```python
from build123d import *

# Parameters (mm, degrees)
SKETCH1_R               = 11
BOSS_EXTRUDE1_DEPTH     = 216.66667
BOSS_EXTRUDE2_START     = 216.66667
SKETCH2_R               = 6.8
BOSS_EXTRUDE2_DEPTH     = 19.8
CUT_EXTRUDE2_START      = -1.4
SKETCH4_R               = 0.5
CUT_EXTRUDE2_DEPTH      = 9
SKETCH6_R               = 7
CUT_EXTRUDE3_DEPTH      = 20
CUT_EXTRUDE4_DEPTH      = 237.977817671
CUT_EXTRUDE4_DEPTH_BACK = 237.977817671
SKETCH7_R               = 0.5
CUT_EXTRUDE5_DEPTH      = 237.97781768
CUT_EXTRUDE5_DEPTH_BACK = 237.97781768
SKETCH10_R              = 0.5
CUT_EXTRUDE6_DEPTH      = 237.97781768
CUT_EXTRUDE6_DEPTH_BACK = 237.97781768
SKETCH11_W              = 2
SKETCH11_H              = 46.680194511
BOSS_EXTRUDE3_START     = 2.5
SKETCH14_R              = 10
BOSS_EXTRUDE3_DEPTH     = 28.5


with BuildPart() as part:
    # Sketch1 → Boss-Extrude1 (new body)
    with BuildSketch(Plane(origin=(0, 0, 0), x_dir=(1, 0, 0), z_dir=(0, 1, 0))):
        with Locations(Location((0, 0, 0), (0, 0, 270))):
            Circle(SKETCH1_R)
    extrude(amount=BOSS_EXTRUDE1_DEPTH)

    # Sketch2 → Boss-Extrude2 (add)
    with BuildSketch(Plane(origin=(0, 0, 0), x_dir=(1, 0, 0), z_dir=(0, 1, 0)).offset(BOSS_EXTRUDE2_START)):
        with Locations(Location((0, 0, 0), (0, 0, 90))):
            Circle(SKETCH2_R)
    extrude(amount=BOSS_EXTRUDE2_DEPTH)

    # Sketch4 → Cut-Extrude2 (cut)
    with BuildSketch(Plane(origin=(0, 0, 0), x_dir=(0, 0, -1), z_dir=(1, 0, 0)).offset(CUT_EXTRUDE2_START)):
        with Locations((0, 226.66667)):
            Circle(SKETCH4_R)
    cut_extrude2 = extrude(amount=-CUT_EXTRUDE2_DEPTH, mode=Mode.SUBTRACT)

    # Mirror2: Cut-Extrude2 across plane
    add(cut_extrude2.mirror(Plane(origin=(0, 0, 0), x_dir=(0, 0, 1), z_dir=(1, 0, 0))), mode=Mode.SUBTRACT)

    # Sketch6 → Cut-Extrude3 (cut)
    with BuildSketch(Plane(origin=(0, 0, 0), x_dir=(1, 0, 0), z_dir=(0, 1, 0))):
        with Locations(Location((0, 0, 0), (0, 0, 270))):
            Circle(SKETCH6_R)
    extrude(amount=CUT_EXTRUDE3_DEPTH, mode=Mode.SUBTRACT)

    # Sketch7 → Cut-Extrude4 (cut, two sides: drawn at the far end of the back side and taken through both)
    with BuildSketch(Plane(origin=(0, 0, 0), x_dir=(0, 0, -1), z_dir=(1, 0, 0)).offset(-CUT_EXTRUDE4_DEPTH_BACK)):
        with Locations((0, 10)):
            Circle(SKETCH7_R)
    extrude(amount=CUT_EXTRUDE4_DEPTH + CUT_EXTRUDE4_DEPTH_BACK, mode=Mode.SUBTRACT)

    # Sketch10 → Cut-Extrude5 (cut, two sides: drawn at the far end of the back side and taken through both)
    with BuildSketch(Plane.XY.offset(-CUT_EXTRUDE5_DEPTH_BACK)):
        with Locations((0, 5)):
            Circle(SKETCH10_R)
    extrude(amount=CUT_EXTRUDE5_DEPTH + CUT_EXTRUDE5_DEPTH_BACK, mode=Mode.SUBTRACT)

    # Sketch11 → Cut-Extrude6 (cut, two sides: drawn at the far end of the back side and taken through both)
    with BuildSketch(Plane.XY.offset(-CUT_EXTRUDE6_DEPTH_BACK)):
        with Locations((0, 213.126572745)):
            Rectangle(SKETCH11_W, SKETCH11_H)
    extrude(amount=CUT_EXTRUDE6_DEPTH + CUT_EXTRUDE6_DEPTH_BACK, mode=Mode.SUBTRACT)

    # Sketch14 → Boss-Extrude3 (add)
    with BuildSketch(Plane(origin=(0, 0, 0), x_dir=(0, 0, -1), z_dir=(1, 0, 0)).offset(BOSS_EXTRUDE3_START)):
        with Locations(Location((0, 160, 0), (0, 0, 180))):
            Circle(SKETCH14_R)
    boss_extrude3 = extrude(amount=BOSS_EXTRUDE3_DEPTH)

    # Mirror3: Boss-Extrude3 across plane
    add(boss_extrude3.mirror(Plane(origin=(0, 0, 0), x_dir=(0, 0, 1), z_dir=(1, 0, 0))))


solid = part.part
```
Input: part model. Units: mm. Frame: model coordinates. A direction names the side the tool comes from. Give positions to 0.01 mm unless a question says otherwise; leave off trailing zeros. Order: outer loops, then holes, each group sorted by start corner. A loop starts at its lowest first (then second) coordinate and runs counter-clockwise, first axis right, second up. Notation, with made-up numbers: M 80,5.25 L 124,5.25 A14 cw 124,26.25 Z; hole C 89.5,60 d7. An arc over 180 degrees is marked long. Return JSON: item names as keys, results as strings.
1) Section query D-D on y = 84. Output: boundary loops of the cut face in (x, z).
Taken from the geometry:
{"outline": "C 0,0 d22"}
2) Section query B-B on y = 213.5. Output: boundary loops of the cut face in (x, z).
Taken from the geometry:
{"outline": "M -1,-10.95 L -1,10.95 A11 ccw Z; M 1,-10.95 A11 ccw 1,10.95 Z"}
3) Line query: L1, parallel to Z at x = 0, y = 11.75; L2, parallel to Y at x = -8, z = 0; L3, parallel to Y at x = -5.2, z = 0. Output: solid intervals per line, ascending. Write a range as [from, to].
Taken from the geometry:
{"L1": "z = [-11, -7], [7, 11]", "L2": "y = [0, 9.5], [10.5, 216.67]", "L3": "y = [20, 226.17], [227.17, 236.47]"}
4) Mould query, pull axis X, two halves, no side actions, for faces 4 (the face through (-4.213, 106.817, 10.161)), 5 (the face through (6.42, 226.43, 2.24)), 6 (the face through (0.2, 0, 7.2)), 7 (the face through (0, 20, 0)). Classes: released by +X, released by -X, zero draft, split by the parting line, or undercut.
Taken from the geometry:
{"face 4": "split by the parting line", "face 5": "released by +X", "face 6": "zero draft", "face 7": "undercut"}
5) Section query C-C on x = -24. Output: boundary loops of the cut face in (y, z).
Taken from the geometry:
{"outline": "C 160,0 d20"}
6) Section query A-A on y = 160. Output: boundary loops of the cut face in (x, z), and give its area (3 significant figures).
Taken from the geometry:
{"outline": "M -31,-10 L -4.58,-10 A11 ccw 4.58,-10 L 31,-10 L 31,10 L 4.58,10 A11 ccw -4.58,10 L -31,10 Z", "area": "1,250 mm2"}
7) Contact query for flat-ended pins moving along their axis: pin 1 (12 mm diameter, centred on x = -14, y = 122, fed in from -Z); pin 2 (12 mm diameter, centred on y = 47.5, z = 7, fed in from +X); pin 3 (4 mm diameter, centred on y = 103.5, z = -3.5, fed in from -X). Output: stop coordinate, or through.
Taken from the geometry:
{"pin 1": "stops at z = -7.55", "pin 2": "stops at x = 10.95", "pin 3": "stops at x = -10.9"}
8) Access query for faces 1 (the face through (-6.834, 9.86, -1.517)), 2 (the face through (7, 216.667, 0)), 3 (the face through (1, 208, 0)). Directions: +Z, -Z, +X, -X, +Y, -Y. A direction counts if a zero-diameter tool reaches every point of the face in a straight line with its end or side. Return the directions, or none.
Taken from the geometry:
{"face 1": "-Y", "face 2": "+X, +Y", "face 3": "+Z, -Z, +Y"}
